Geometry check sheet. Reference: drawing and pictorial views, mm from the part's lowest x, y, z. A direction names the side the tool comes from. Round coordinates to 2 decimals unless told otherwise and drop trailing zeros. Loops run counter-clockwise (first coordinate to the right, second up) from the corner with the lowest first, then second, coordinate; pieces in that order, holes last. Notation, with made-up numbers: M -0.5,49 L 13.5,49 A9 cw 13.5,54 Z; hole C 18,-9 d10. An arc over 180 degrees is marked long. One line per question, with ' | ' between items. Start each with the question number.
(1) Go/stop test with flat-tipped pins: P1, Ø2.5, axis at y = 26.5, z = 6.5, coming from the -X side; P2, Ø2, axis at y = 49, z = 1, coming from the +X side; P3, Ø1, axis at y = 47.5, z = 4.5, coming from the -X side; P4, Ø3, axis at x = 7.5, z = 6, coming from the -Y side. Record where each tip stops, or that it passes through.
(2) Tool access check on the marked faces 1 and 2. Record the directions out of +Z, -Z, +X, -X, +Y, -Y that give a thin tool (end or side, any length) a straight path to the whole face; none if there is none.
(3) Section check A-A (z = 5.75). Record the boundary of the cut face in (x, y).
(4) Thickness scan on probe 1 along X at (y, z) = (43, 0.5); probe 2 along X at (y, z) = (45.5, 7); probe 3 along Z at (x, y) = (29, 54.5). Record the ranges inside material, lowest first. Write a range as [from, to].
(5) Draft check along Y on the marked faces 3, 4, 5 and 6. Enter one of: +Y half, -Y half, draft (parallel to the pull), parting line (faces both ways), or undercut.
(6) Section check B-B (z = 1.25). Record the boundary of the cut face in (x, y), and give its area (3 significant figures).
(7) Section check C-C (y = 43.5). Record the boundary of the cut face in (x, z), and give its area (3 significant figures).
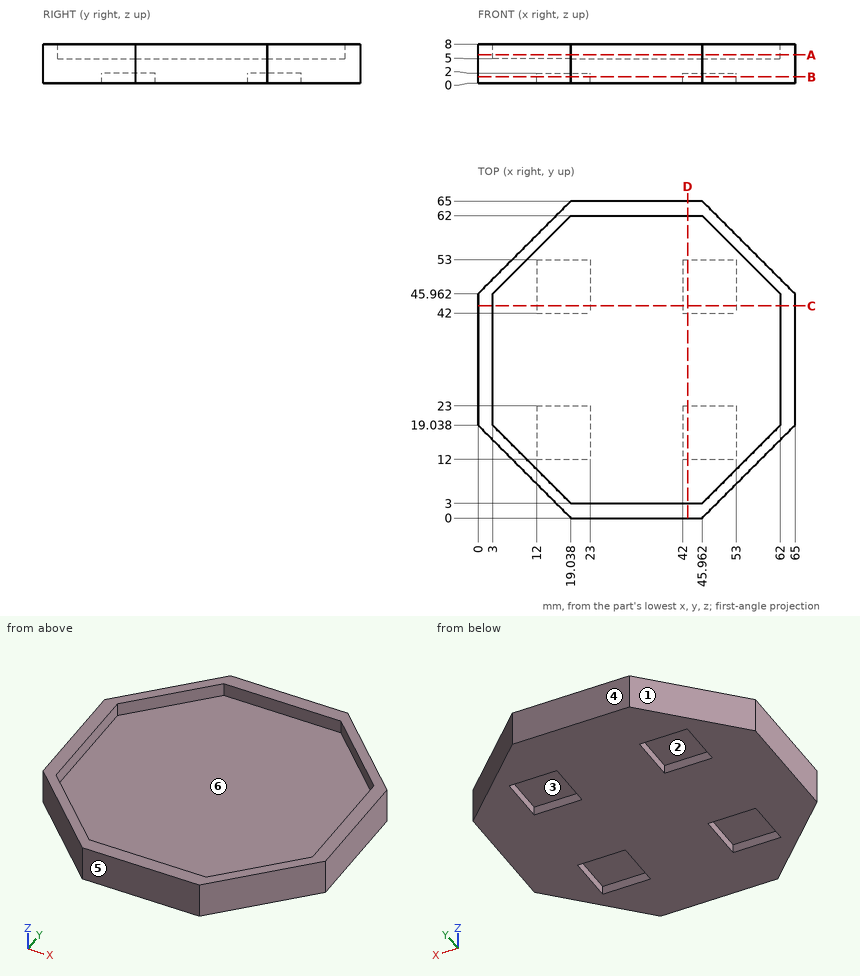
The answers:
1) P1: x = 0 | P2: x = 62.96 | P3: x = 1.04 | P4: y = 10.04
2) face 1: +Z, -Z, -X, +Y | face 2: -Z
3) outline: M 0,19.04 L 19.04,0 L 45.96,0 L 65,19.04 L 65,45.96 L 45.96,65 L 19.04,65 L 0,45.96 Z; hole M 3,19.04 L 19.04,3 L 45.96,3 L 62,19.04 L 62,45.96 L 45.96,62 L 19.04,62 L 3,45.96 Z
4) probe 1: [0, 12], [23, 42], [53, 65] | probe 2: [0, 3], [62, 65] | probe 3: [0, 5]
5) face 3: undercut | face 4: +Y half | face 5: -Y half | face 6: undercut
6) outline: M 0,19.04 L 19.04,0 L 45.96,0 L 65,19.04 L 65,45.96 L 45.96,65 L 19.04,65 L 0,45.96 Z; hole M 12,12 L 23,12 L 23,23 L 12,23 Z; hole M 12,42 L 23,42 L 23,53 L 12,53 Z; hole M 42,12 L 53,12 L 53,23 L 42,23 Z; hole M 42,42 L 53,42 L 53,53 L 42,53 Z | area: 3,020 mm²
7) outline: M 0,0 L 12,0 L 12,2 L 23,2 L 23,0 L 42,0 L 42,2 L 53,2 L 53,0 L 65,0 L 65,8 L 62,8 L 62,5 L 3,5 L 3,8 L 0,8 Z | area: 299 mm²
